Model file for the job. Use its own axes, mm. Round coordinates to 2 decimals unless told otherwise and drop trailing zeros. Loops run counter-clockwise (first coordinate to the right, second up) from the corner with the lowest first, then second, coordinate; pieces in that order, holes last. Notation, with made-up numbers: M 53.5,6 L 66.5,6 A6 ccw 66.5,10 Z; hole C -7,34.5 d5. An arc over 180 degrees is marked long. Use a Markdown table: item, result. Add a question column.
Item 1: Saw through at C-C on y = 33.3. Give the number of separate pieces and of enclosed holes in the cut face, then the cut area to 3 significant figures.
Item 2: Pin check, flat tips, straight feed: P1, Ø0.9, axis at x = -18, y = 34.5, coming from the +Z side; P2, Ø0.9, axis at y = 34.5, z = -135, coming from the -X side; P3, Ø0.9, axis at x = -24.5, y = 34.5, coming from the -Z side; P4, Ø1.5, axis at x = 14.5, z = -101.5, coming from the +Y side. Stop position of each tip, or through.
Item 3: Saw through at D-D on x = -2.5. Write the cut outline in (y, z).
Item 4: Saw through at B-B on z = -137.5. Write the cut outline in (x, y), then the cut area to 3 significant figures.
Item 5: Wall check: L1, parallel to Z at x = -5, y = 34.4; L2, parallel to Z at x = -22.5, y = 33.3; L3, parallel to Z at x = 4.5, y = 33.9. Give the ranges that are in metal, low to high. Write a range as from..to.
Item 6: Saw through at A-A on x = 17. Write the cut outline in (y, z).
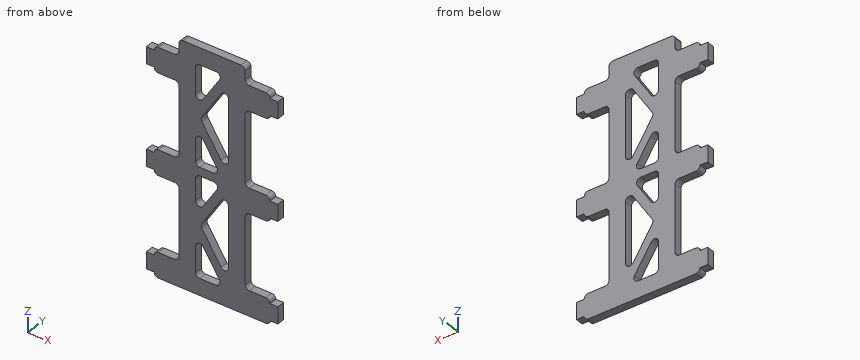
```python
from build123d import *

# Parameters (mm, degrees)
SKETCH1_W           = 25.4
SKETCH1_H           = 92.075
BOSS_EXTRUDE1_DEPTH = 1.5
SKETCH2_W           = 9.525
SKETCH2_H           = 9.525
BOSS_EXTRUDE2_DEPTH = 3
CUT_EXTRUDE1_DEPTH  = 169.189397054
FILLET1_R           = 1.5875
SKETCH5_W           = 3
SKETCH5_H           = 6.35
BOSS_EXTRUDE3_DEPTH = 3


with BuildPart() as part:
    # Sketch1 → Boss-Extrude1 (new, symmetric)
    with BuildSketch(Plane(origin=(0, 34.29, 0), x_dir=(1, 0, 0), z_dir=(0, 1, 0))):
        with Locations((0, 120.65)):
            Rectangle(SKETCH1_W, SKETCH1_H)
    extrude(amount=BOSS_EXTRUDE1_DEPTH, both=True)

    # Sketch2 → Boss-Extrude2 (add)
    with BuildSketch(Plane(origin=(0, 35.79, 0), x_dir=(1, 0, 0), z_dir=(0, 1, 0))):
        with Locations((17.4625, 161.925)):
            Rectangle(SKETCH2_W, SKETCH2_H)
        with Locations((-17.4625, 161.925)):
            Rectangle(SKETCH2_W, SKETCH2_H)
        with Locations((17.4625, 123.825)):
            Rectangle(SKETCH2_W, SKETCH2_H)
        with Locations((-17.4625, 123.825)):
            Rectangle(SKETCH2_W, SKETCH2_H)
        with Locations((17.4625, 85.725)):
            Rectangle(SKETCH2_W, SKETCH2_H)
        with Locations((-17.4625, 85.725)):
            Rectangle(SKETCH2_W, SKETCH2_H)
    extrude(amount=-BOSS_EXTRUDE2_DEPTH)

    # Sketch4 → Cut-Extrude1 (cut, through all)
    with BuildSketch(Plane(origin=(0, 35.79, 0), x_dir=(1, 0, 0), z_dir=(0, 1, 0))):
        Polygon((4.465215596, 80.9625), (-6.35, 97.861274369), (-6.35, 80.9625), align=None)
        Polygon((6.35, 83.907475631), (6.35, 117.705024369), (-4.465215596, 100.80625), align=None)
        Polygon((3.449215596, 119.0625), (-6.35, 119.0625), (-6.35, 103.751225631), align=None)
        Polygon((3.449215596, 122.2375), (-6.35, 137.548774369), (-6.35, 122.2375), align=None)
        Polygon((6.35, 123.594975631), (6.35, 157.392524369), (-4.465215596, 140.49375), align=None)
        Polygon((4.465215596, 160.3375), (-6.35, 160.3375), (-6.35, 143.438725631), align=None)
    extrude(amount=-CUT_EXTRUDE1_DEPTH, mode=Mode.SUBTRACT)

    # Fillet1
    fillet1_edges = [part.edges().sort_by_distance(p)[0] for p in [
        (3.449215596, 34.29, -119.0625),
        (-6.35, 34.29, -103.751225631),
        (-6.35, 34.29, -119.0625),
        (-4.465215596, 34.29, -100.80625),
        (6.35, 34.29, -117.705024369),
        (6.35, 34.29, -83.907475631),
        (-4.465215596, 34.29, -140.49375),
        (6.35, 34.29, -157.392524369),
        (6.35, 34.29, -123.594975631),
        (3.449215596, 34.29, -122.2375),
        (-6.35, 34.29, -122.2375),
        (-6.35, 34.29, -137.548774369),
        (-6.35, 34.29, -143.438725631),
        (-6.35, 34.29, -160.3375),
        (4.465215596, 34.29, -160.3375),
        (4.465215596, 34.29, -80.9625),
        (-6.35, 34.29, -80.9625),
        (-6.35, 34.29, -97.861274369),
        (22.225, 34.29, -80.9625),
        (22.225, 34.29, -90.4875),
        (12.7, 34.29, -90.4875),
        (12.7, 34.29, -80.9625),
        (-12.7, 34.29, -119.0625),
        (-12.7, 34.29, -128.5875),
        (-22.225, 34.29, -128.5875),
        (-22.225, 34.29, -119.0625),
        (22.225, 34.29, -119.0625),
        (22.225, 34.29, -128.5875),
        (12.7, 34.29, -128.5875),
        (12.7, 34.29, -119.0625),
        (-12.7, 34.29, -157.1625),
        (-22.225, 34.29, -166.6875),
        (-22.225, 34.29, -157.1625),
        (-12.7, 34.29, -80.9625),
        (-12.7, 34.29, -90.4875),
        (-22.225, 34.29, -90.4875),
        (-22.225, 34.29, -80.9625),
        (22.225, 34.29, -157.1625),
        (22.225, 34.29, -166.6875),
        (12.7, 34.29, -157.1625),
        (-12.7, 34.29, -74.6125),
        (12.7, 34.29, -74.6125),
    ]]
    fillet(fillet1_edges, radius=FILLET1_R)

    # Sketch5 → Boss-Extrude3 (add)
    with BuildSketch(Plane(origin=(0, 35.79, 0), x_dir=(1, 0, 0), z_dir=(0, 1, 0))):
        with Locations((23.725, 161.925)):
            Rectangle(SKETCH5_W, SKETCH5_H)
        with Locations((-23.725, 161.925)):
            Rectangle(SKETCH5_W, SKETCH5_H)
        with Locations((23.725, 123.825)):
            Rectangle(SKETCH5_W, SKETCH5_H)
        with Locations((-23.725, 123.825)):
            Rectangle(SKETCH5_W, SKETCH5_H)
        with Locations((23.725, 85.725)):
            Rectangle(SKETCH5_W, SKETCH5_H)
        with Locations((-23.725, 85.725)):
            Rectangle(SKETCH5_W, SKETCH5_H)
    extrude(amount=-BOSS_EXTRUDE3_DEPTH)


solid = part.part
```
Entries:
| question | item | result |
|---|---|---|
| 1 | separate pieces | 1 |
| 1 | enclosed holes | 6 |
| 1 | area | 2,350 mm2 |
| 2 | P1 | z = -80.96 |
| 2 | P2 | x = -12.7 |
| 2 | P3 | z = -165.1 |
| 2 | P4 | through |
| 3 | outline | M 32.79,-166.69 L 35.79,-166.69 L 35.79,-160.34 L 32.79,-160.34 Z; M 32.79,-149.45 L 35.79,-149.45 L 35.79,-143.56 L 32.79,-143.56 Z; M 32.79,-137.42 L 35.79,-137.42 L 35.79,-131.53 L 32.79,-131.53 Z; M 32.79,-122.24 L 35.79,-122.24 L 35.79,-119.06 L 32.79,-119.06 Z; M 32.79,-109.77 L 35.79,-109.77 L 35.79,-103.88 L 32.79,-103.88 Z; M 32.79,-97.74 L 35.79,-97.74 L 35.79,-91.85 L 32.79,-91.85 Z; M 32.79,-80.96 L 35.79,-80.96 L 35.79,-74.61 L 32.79,-74.61 Z |
| 4 | outline | M -12.7,32.79 L -2.55,32.79 L -2.55,35.79 L -12.7,35.79 Z; M 6.35,32.79 L 12.7,32.79 L 12.7,35.79 L 6.35,35.79 Z |
| 4 | area | 49.5 mm2 |
| 5 | L1 | -166.69..-160.32, -147.29..-133.69, -122.26..-119.04, -107.61..-94.01, -80.98..-74.61 |
| 5 | L2 | -165.1..-158.75, -127..-120.65, -88.9..-82.55 |
| 5 | L3 | -166.69..-153.53, -127.45..-113.85, -87.77..-74.61 |
| 6 | outline | M 32.79,-166.69 L 35.79,-166.69 L 35.79,-157.16 L 32.79,-157.16 Z; M 32.79,-128.59 L 35.79,-128.59 L 35.79,-119.06 L 32.79,-119.06 Z; M 32.79,-90.49 L 35.79,-90.49 L 35.79,-80.96 L 32.79,-80.96 Z |
